from build123d import *

# Parameters (mm, degrees)
SKETCH_1_R          = 11
EXTRUDE_1_DEPTH     = 3
SKETCH_2_R          = 5
EXTRUDE_2_DEPTH     = 12
SKETCH_5_R          = 1.6
CUT_EXTRUDE_3_DEPTH = 4
FILLET_1_R          = 0.35
SKETCH_7_R          = 5
EXTRUDE_3_DEPTH     = 1.5
HOLE_WIZARD_M8_1_D  = 6.8


with BuildPart() as part:
    # 草图1 → 凸台-拉伸1 (new body)
    with BuildSketch(Plane(origin=(0, 0, 0), x_dir=(1, 0, 0), z_dir=(0, 1, 0))):
        Circle(SKETCH_1_R)
    extrude(amount=EXTRUDE_1_DEPTH)

    # 草图2 → 凸台-拉伸2 (add)
    with BuildSketch(Plane(origin=(0, 3, 0), x_dir=(1, 0, 0), z_dir=(0, 1, 0))):
        Circle(SKETCH_2_R)
    extrude(amount=EXTRUDE_2_DEPTH)

    # 草图5 → 切除-拉伸3 (cut, through all)
    with BuildSketch(Plane(origin=(0, 3, 0), x_dir=(1, 0, 0), z_dir=(0, 1, 0))):
        with Locations((0, 8)):
            Circle(SKETCH_5_R)
        with Locations((8, 0)):
            Circle(SKETCH_5_R)
        with Locations((0, -8)):
            Circle(SKETCH_5_R)
        with Locations((-8, 0)):
            Circle(SKETCH_5_R)
    extrude(amount=-CUT_EXTRUDE_3_DEPTH, mode=Mode.SUBTRACT)

    # 圆角1
    fillet_1_edges = [part.edges().sort_by_distance(p)[0] for p in [
        (-5, 15, 0),
    ]]
    fillet(fillet_1_edges, radius=FILLET_1_R)

    # 草图7 → 凸台-拉伸3 (add)
    with BuildSketch(Plane.XZ):
        Circle(SKETCH_7_R)
    extrude(amount=EXTRUDE_3_DEPTH)

    # M8 螺纹孔1 (through all)
    with Locations(Plane(origin=(0, 15, 0), x_dir=(1, 0, 0), z_dir=(0, 1, 0))):
        with Locations((0, 0)):
            Hole(HOLE_WIZARD_M8_1_D / 2)


solid = part.part
Verification items for the finished model (mm, model axes). A direction names the side the tool comes from. Round coordinates to 2 decimals unless told otherwise and drop trailing zeros. Loops run counter-clockwise (first coordinate to the right, second up) from the corner with the lowest first, then second, coordinate; pieces in that order, holes last. Notation, with made-up numbers: (60.25, -16.75) - (96.25, -16.75) arc R13 ccw to (96.25, -11.75) - close; hole circle Ø3 at (-3.5, 79). An arc over 180 degrees is marked (long way). Answer in a Markdown table with one row per item. Add a question column.
Q1. Gauge pin test, flat ends, axial feed: pin 1 (6 mm diameter, centred on x = -8.5, y = 3.5, fed in from -Z); pin 2 (4 mm diameter, centred on x = -8, z = 0, fed in from -Y); pin 3 (2 mm diameter, centred on y = 11, z = -3, fed in from +X). Record the tip position at first contact, or that the pin passes through.
Q2. Material ranges on line 1 (Z direction, x = 0, y = 2.15); line 2 (Z direction, x = 0, y = 11.25); line 3 (Z direction, x = 0.75, y = 1.75), recorded low to high.
Q3. Release check for a two-part mould opening along Z. For faces 3 (the face through (-0.35, 1.52, 9.56)), 4 (the face through (-1.08, -0.74, -4.88)), 5 (the face through (5, 0, 2)) record: pulls with the +Z half, pulls with the -Z half, needs draft (parallel to the pull), parting line crosses it, or undercut.
Q4. Section check B-B on y = 0.75. Enter the section's corners in (x, z), plus the area to 3 significant figures.
Q5. Section check C-C on z = 0. Enter the section's corners in (x, y).
Q6. Tool access check on faces 1 (the face through (0.74, 6.63, 3.32)), 2 (the face through (-1.08, 8.74, 4.88)). Record the directions out of +Z, -Z, +X, -X, +Y, -Y that give a thin tool (end or side, any length) a straight path to the whole face; none if there is none.
Q7. Section check A-A on x = 0. Enter the section's corners in (y, z).
Q8. Section check D-D on x = 8.5. Enter the section's corners in (y, z), plus the area to 3 significant figures.
Found:
| question | item | result |
|---|---|---|
| 1 | pin 1 | stops at z = -9.5 |
| 1 | pin 2 | stops at y = 0 |
| 1 | pin 3 | stops at x = 4.58 |
| 2 | line 1 | z = -11 to -9.6, -6.4 to -3.4, 3.4 to 6.4, 9.6 to 11 |
| 2 | line 2 | z = -5 to -3.4, 3.4 to 5 |
| 2 | line 3 | z = -10.97 to -9.41, -6.59 to -3.32, 3.32 to 6.59, 9.41 to 10.97 |
| 3 | face 3 | undercut |
| 3 | face 4 | parting line crosses it |
| 3 | face 5 | needs draft |
| 4 | outline | circle Ø22 at (0, 0); hole circle Ø3.2 at (-8, 0); hole circle Ø6.8 at (0, 0); hole circle Ø3.2 at (0, -8); hole circle Ø3.2 at (0, 8); hole circle Ø3.2 at (8, 0) |
| 4 | area | 312 mm² |
| 5 | outline | (-11, 0) - (-9.6, 0) - (-9.6, 3) - (-11, 3) - close; (-6.4, 0) - (-5, 0) - (-5, -1.5) - (-3.4, -1.5) - (-3.4, 15) - (-4.65, 15) arc R0.35 ccw to (-5, 14.65) - (-5, 3) - (-6.4, 3) - close; (3.4, -1.5) - (5, -1.5) - (5, 0) - (6.4, 0) - (6.4, 3) - (5, 3) - (5, 14.65) arc R0.35 ccw to (4.65, 15) - (3.4, 15) - close; (9.6, 0) - (11, 0) - (11, 3) - (9.6, 3) - close |
| 6 | face 1 | +Y, -Y |
| 6 | face 2 | +Y |
| 7 | outline | (-1.5, -5) - (0, -5) - (0, -6.4) - (3, -6.4) - (3, -5) - (14.65, -5) arc R0.35 ccw to (15, -4.65) - (15, -3.4) - (-1.5, -3.4) - close; (-1.5, 3.4) - (15, 3.4) - (15, 4.65) arc R0.35 ccw to (14.65, 5) - (3, 5) - (3, 6.4) - (0, 6.4) - (0, 5) - (-1.5, 5) - close; (0, -11) - (3, -11) - (3, -9.6) - (0, -9.6) - close; (0, 9.6) - (3, 9.6) - (3, 11) - (0, 11) - close |
| 8 | outline | (0, -6.98) - (3, -6.98) - (3, -1.52) - (0, -1.52) - close; (0, 1.52) - (3, 1.52) - (3, 6.98) - (0, 6.98) - close |
| 8 | area | 32.8 mm² |
